Verification items for the finished model (mm, model axes). A direction names the side the tool comes from. Coordinates: 2 decimals unless noted, no trailing zeros. Order: outer loops, then holes, each group sorted by start corner. A loop starts at its lowest first (then second) coordinate and runs counter-clockwise, first axis right, second up.
Q1. Thickness scan on line 1 (X direction, y = 22, z = -0.25); line 2 (X direction, y = 36, z = 3.5). Record the ranges inside material, lowest first.
Q2. Set-up check for faces 1 (the flat face through (0, 40, 1)), 2 (the flat face through (2.755, 26.947, 1.817)): record each of +Z, -Z, +X, -X, +Y, -Y from which the full face is reachable in a straight line by a thin tool's end or side.
Q3. Depth check by flat-ended pin: P1, Ø2, axis at x = -2.5, y = 17, coming from the -Z side. Enter the tip coordinate at first touch or a pass-through.
Q4. Cross-section at B-B, the plane y = 10.5. Record the boundary of the cut face in (x, z), and give its area (3 significant figures).
Q5. Cross-section at A-A, the plane y = 37. Record the boundary of the cut face in (x, z).
from build123d import *

# Parameters (mm, degrees)
SKETCH1_R           = 4
BOSS_EXTRUDE1_DEPTH = 40
FILLET1_R           = 1
CUT_EXTRUDE1_START  = -25.7
CUT_EXTRUDE1_DEPTH  = 25.7
SKETCH3_R           = 0.05
CUT_EXTRUDE2_DEPTH  = 0.1


with BuildPart() as part:
    # Sketch1 → Boss-Extrude1 (new body)
    with BuildSketch(Plane(origin=(0, 0, 0), x_dir=(1, 0, 0), z_dir=(0, 1, 0))):
        with Locations(Location((0, 0, 0), (0, 0, 270))):
            Circle(SKETCH1_R)
    extrude(amount=BOSS_EXTRUDE1_DEPTH)

    # Fillet1
    fillet1_edges = [part.edges().sort_by_distance(p)[0] for p in [
        (0, 40, -4),
    ]]
    fillet(fillet1_edges, radius=FILLET1_R)

    # Sketch2 → Cut-Extrude1 (cut)
    with BuildSketch(Plane(origin=(0, 40, 0), x_dir=(1, 0, 0), z_dir=(0, 1, 0)).offset(CUT_EXTRUDE1_START)):
        with BuildLine():
            Line((1.546188852, -3.68907848), (3.998512047, 0.109093573))
            ThreePointArc((3.998512047, 0.109093573), (3.360424787, -2.169687823), (1.546188852, -3.68907848))
        make_face()
    extrude(amount=CUT_EXTRUDE1_DEPTH, mode=Mode.SUBTRACT)

    # Sketch3 → Cut-Extrude2 (cut)
    with BuildSketch(Plane(origin=(0, 40, 0), x_dir=(1, 0, 0), z_dir=(0, 1, 0))):
        with Locations(Location((0, 0, 0), (0, 0, 270))):
            Circle(SKETCH3_R)
    extrude(amount=-CUT_EXTRUDE2_DEPTH, mode=Mode.SUBTRACT)


solid = part.part
Check values:
1. line 1: x = -3.99 to 3.99
1. line 2: x = -1.94 to 1.67
2. face 1: +Z, -Z, +X, -X, +Y
2. face 2: +Z, +X, +Y
3. P1: stops at z = -3.71
4. outline: circle Ø8 at (0, 0)
4. area: 50.3 mm2
5. outline: (1.55, 3.69) arc R4 ccw (long way) to (4, -0.11) - close
